For this review, take the finished solid that the model builds, in its own axes (mm). Give positions to 0.01 mm unless a question says otherwise; leave off trailing zeros. Write each loop counter-clockwise with the first axis right and the second up, starting at its lowest first coordinate (ties: lowest second). Pieces come first, ordered by that corner, then holes.
Q1. Insertion check: P1, Ø5, axis at y = -1, z = 177.5, coming from the +X side; P2, Ø1, axis at x = 4, y = 7, coming from the +Z side; P3, Ø6, axis at x = 1.5, z = 152, coming from the +Y side. Each pin has a flat end and moves straight along its axis. Give the tip position at first contact, or say it passes through.
Q2. We need section C-C (z = 101). Write out the cut boundary in (x, y).
Q3. For line 1 (Z direction, x = -10, y = -1.5); line 2 (Z direction, x = 5.25, y = 3.75); line 3 (Z direction, x = 3, y = 2), list the stretches that pass through material, from the lowest coordinate up.
```python
from build123d import *

# Parameters (mm, degrees)
F0_R      = 11.1125
F1_DEPTH  = 1.5875
F2_R      = 9.525
F3_DEPTH  = 3.175
F4_R      = 11.1125
F5_DEPTH  = 1.5875
F6_R      = 6.35
F7_DEPTH  = 2.38125
F8_R      = 4.7625
F9_DEPTH  = 7.112
F10_R     = 2.15265
F11_DEPTH = 203.2


with BuildPart() as f1:
    # F0 (on Top) → F1 (new body)
    with BuildSketch(Plane.XY):
        Circle(F0_R)
    extrude(amount=F1_DEPTH)

    # F2 (on face) → F3 (join)
    with BuildSketch(Plane.XY.offset(1.5875)):
        Circle(F2_R)
    extrude(amount=F3_DEPTH)

    # F4 (on face) → F5 (join)
    with BuildSketch(Plane.XY.offset(4.7625)):
        Circle(F4_R)
    extrude(amount=F5_DEPTH)

    # F6 (on face) → F7 (join)
    with BuildSketch(Plane.XY.offset(6.35)):
        Circle(F6_R)
    extrude(amount=F7_DEPTH)

    # F8 (on face) → F9 (join)
    with BuildSketch(Plane.XY.offset(8.73125)):
        Circle(F8_R)
    extrude(amount=F9_DEPTH)

    # F10 (on face) → F11 (join)
    with BuildSketch(Plane.XY.offset(15.84325)):
        Circle(F10_R)
    extrude(amount=F11_DEPTH)


solid = f1.part
```
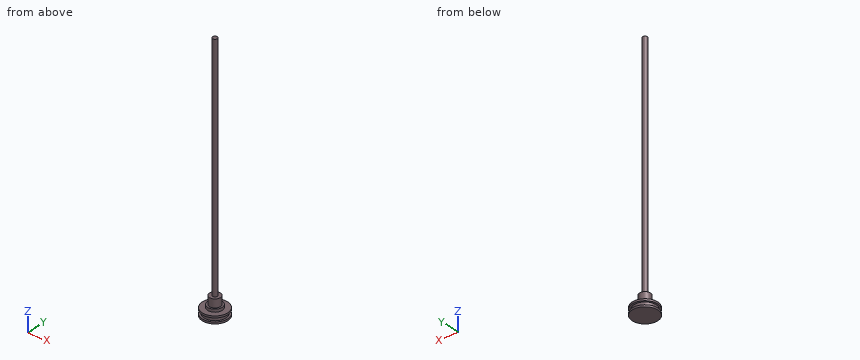
Computed:
1. P1: stops at x = 2.15
1. P2: stops at z = 6.35
1. P3: stops at y = 2.15
2. outline: circle Ø4.31 at (0, 0)
3. line 1: z = 0 to 1.59, 4.76 to 6.35
3. line 2: z = 0 to 6.35
3. line 3: z = 0 to 15.84
